Input: part model. Units: mm. Frame: model coordinates. Round coordinates to 2 decimals unless told otherwise and drop trailing zeros. Write each loop counter-clockwise with the first axis right and the second up, starting at its lowest first coordinate (ties: lowest second). Pieces come first, ordered by that corner, then holes. Notation, with made-up numbers: (57.25, -17.75) - (82.25, -17.75) arc R31 ccw to (82.25, 6.25) - close; hole circle Ø8 at (48.25, -37.75). An arc over 180 degrees is marked (long way). Use one line per item in the form item = value.
```python
from build123d import *

# Parameters (mm, degrees)
SKETCH1_W           = 20
SKETCH1_H           = 20
SKETCH1_W_2         = 18
SKETCH1_H_2         = 18
BOSS_EXTRUDE1_DEPTH = 1240
SKETCH2_R           = 3
CUT_EXTRUDE1_DEPTH  = 1240


with BuildPart() as part:
    # Sketch1 → Boss-Extrude1 (new body)
    with BuildSketch(Plane(origin=(0, 0, 0), x_dir=(0, 0, -1), z_dir=(1, 0, 0))):
        Rectangle(SKETCH1_W, SKETCH1_H)
        Rectangle(SKETCH1_W_2, SKETCH1_H_2, mode=Mode.SUBTRACT)
    extrude(amount=BOSS_EXTRUDE1_DEPTH)

    # Sketch2 → Cut-Extrude1 (cut)
    with BuildSketch(Plane(origin=(0, 10, 0), x_dir=(1, 0, 0), z_dir=(0, 1, 0))):
        with Locations((12, 0)):
            Circle(SKETCH2_R)
        with Locations((24, 0)):
            Circle(SKETCH2_R)
        with Locations((1216, 0)):
            Circle(SKETCH2_R)
        with Locations((1228, 0)):
            Circle(SKETCH2_R)
        with Locations((324, 0)):
            Circle(SKETCH2_R)
        with Locations((312, 0)):
            Circle(SKETCH2_R)
        with Locations((916, 0)):
            Circle(SKETCH2_R)
        with Locations((928, 0)):
            Circle(SKETCH2_R)
    extrude(amount=-CUT_EXTRUDE1_DEPTH, mode=Mode.SUBTRACT)


solid = part.part
```
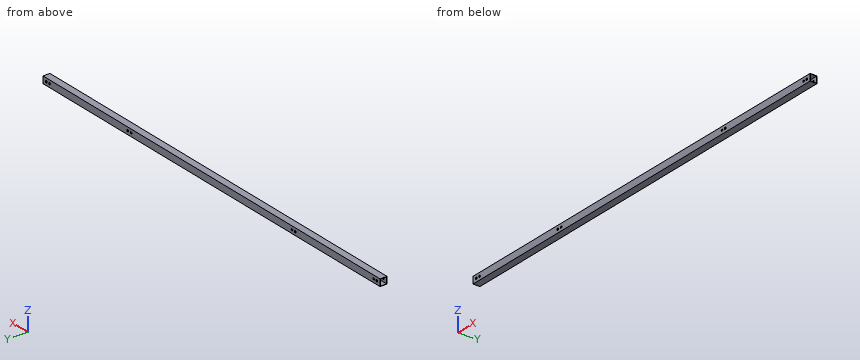
(1) Cut plane A-A on y = -5. Output: boundary loops of the cut face in (x, z), then the cut area to 3 significant figures.
Derived:
outline = (0, -10) - (1240, -10) - (1240, -9) - (0, -9) - close; (0, 9) - (1240, 9) - (1240, 10) - (0, 10) - close
area = 2,480 mm^2
(2) Material intervals for L1, parallel to Y at x = 77, z = 0; L2, parallel to Z at x = 312, y = -9.3, sorted ascending.
Derived:
L1 = -10 to -9, 9 to 10
L2 = -10 to -3, 3 to 10
(3) Cut plane C-C on z = 0. Count the separate pieces of the cut face and the enclosed holes in it, then the cut area to 3 significant figures.
Derived:
separate_pieces = 18
enclosed_holes = 0
area = 2,380 mm^2
(4) Cut plane B-B on x = 697. Output: boundary loops of the cut face in (y, z).
Derived:
outline = (-10, -10) - (10, -10) - (10, 10) - (-10, 10) - close; hole (-9, -9) - (9, -9) - (9, 9) - (-9, 9) - close
